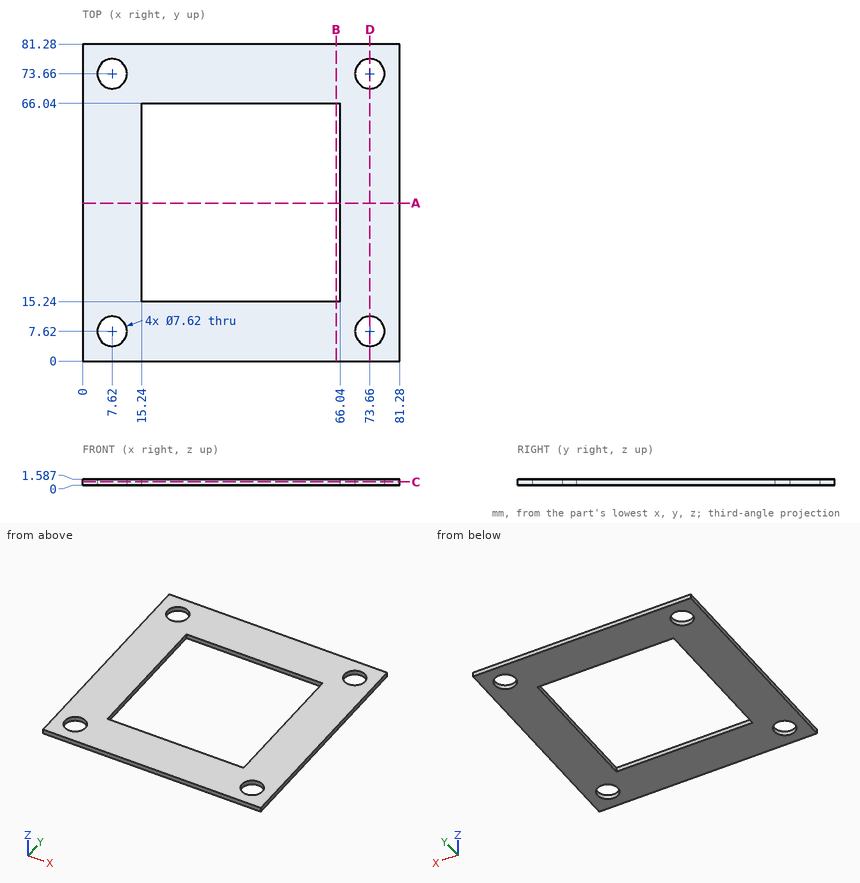
Answer from the drawing. Dimensions are ordinates in mm from the lowest x, y and z of the part. Round coordinates to 2 decimals unless told otherwise and drop trailing zeros. Loops run counter-clockwise (first coordinate to the right, second up) from the corner with the lowest first, then second, coordinate; pieces in that order, holes last. Notation, with made-up numbers: (32.5, 68.25) - (54.5, 68.25) arc R19 cw to (54.5, 89.25) - close; hole circle Ø7 at (14, 62.25). An arc over 180 degrees is marked (long way). Return JSON: item names as keys, results as strings. Group by question number.
1. The part is cut by section C-C on z = 0.85. Determine the outline of the cut face in (x, y).
2. The part is cut by section D-D on x = 73.66. Determine the outline of the cut face in (y, z), then the cut area to 3 significant figures.
3. This flat-tipped pin is pushed along its axis until it touches: P1, Ø4.5, axis at x = 7.62, y = 73.66, coming from the +Z side. Where does it stop, or does it pass through?
4. The part is cut by section A-A on y = 40.5. Determine the outline of the cut face in (x, z).
5. Consider probe 1 along Y at (x, z) = (73.66, 1); probe 2 along Y at (x, z) = (20.5, 1.2). Determine where each line is inside the solid, lowest interval first.
Resolved:
{
 "1": {"outline": "(0, 0) - (81.28, 0) - (81.28, 81.28) - (0, 81.28) - close; hole circle Ø7.62 at (7.62, 7.62); hole circle Ø7.62 at (7.62, 73.66); hole (15.24, 15.24) - (66.04, 15.24) - (66.04, 66.04) - (15.24, 66.04) - close; hole circle Ø7.62 at (73.66, 7.62); hole circle Ø7.62 at (73.66, 73.66)"},
 "2": {"outline": "(0, 0) - (3.81, 0) - (3.81, 1.59) - (0, 1.59) - close; (11.43, 0) - (69.85, 0) - (69.85, 1.59) - (11.43, 1.59) - close; (77.47, 0) - (81.28, 0) - (81.28, 1.59) - (77.47, 1.59) - close", "area": "105 mm²"},
 "3": {"P1": "passes through"},
 "4": {"outline": "(0, 0) - (15.24, 0) - (15.24, 1.59) - (0, 1.59) - close; (66.04, 0) - (81.28, 0) - (81.28, 1.59) - (66.04, 1.59) - close"},
 "5": {"probe 1": "y = 0 to 3.81, 11.43 to 69.85, 77.47 to 81.28", "probe 2": "y = 0 to 15.24, 66.04 to 81.28"}
}
